Build history of the part. All positions in model axes, mm. A direction names the side the tool comes from. Round coordinates to 2 decimals unless told otherwise and drop trailing zeros. Order: outer loops, then holes, each group sorted by start corner. A loop starts at its lowest first (then second) coordinate and runs counter-clockwise, first axis right, second up. Notation, with made-up numbers: (28, 43.5) -> (41, 43.5) arc R31 ccw to (41, 72.5) -> close; hole circle Ø8 at (3, -35). An arc over 180 degrees is marked (long way). Use a Markdown table: item, result. Add a question column.
Item 1: Pin check, flat tip, straight feed: pin 1 (5 mm diameter, centred on x = 0, z = 0, fed in from -Y). Stop position of the tip, or through.
Item 2: 3-axis set-ups, long thin cutter, end or side, ignore diameter. For faces 4 (the face through (-16.9, -4.57, 0.18)), 5 (the face through (-1.86, -19.454, -7.746)): which of +Z, -Z, +X, -X, +Y, -Y reach the whole face in a straight line?
Item 3: Probe L1, parallel to Z at x = 0, y = -11; L2, parallel to X at y = -5, z = 5; L3, parallel to X at y = -6, z = -2.75. List the from-to ranges inside material, lowest first.
Item 4: Slice it at D-D, the plane x = -14. Give the cut face in (y, z), plus the area to 3 significant figures.
Item 5: Slice it at B-B, the plane y = -7. Give the cut face in (x, z), plus the area to 3 significant figures.
Item 6: Slice it at A-A, the plane z = 2.75. Give the cut face in (x, y).
Item 7: Slice it at C-C, the plane z = -10. Give the cut face in (x, y), plus the area to 3 significant figures.
Item 8: Two-plate mould, pull along X, no slides. Class faces 1 (the face through (0.61, -18.95, 8.21)), 2 (the face through (0, -10, -12.5)), 3 (the face through (-17.5, -8, 0)): released by +X, released by -X, zero draft, split by the parting line, or undercut.
from build123d import *

# Parameters (mm, degrees)
PAD_DEPTH         = 12.5
SKETCH001_R       = 4
POCKET_DEPTH      = 0.001
POCKET_DEPTH_BACK = -19.523712


with BuildPart() as part:
    # Sketch → Pad (new body, symmetric)
    with BuildSketch(Plane.XY):
        with BuildLine():
            ThreePointArc((-17.222222, -10.168336), (-11.903544, -16.07189), (-4.705882, -19.438484))
            ThreePointArc((-4.705882, -19.438484), (-4.355445, -19.50158), (-4, -19.522712))
            Line((-4, -19.522712), (-2.5, -19.522712))
            ThreePointArc((-2.5, -19.522712), (-1.850681, -19.4516), (-1.232145, -19.241635))
            Line((-1.232145, -19.241635), (0, -18.667076))
            Line((0, -18.667076), (1.232145, -19.241635))
            ThreePointArc((1.232145, -19.241635), (1.850681, -19.4516), (2.5, -19.522712))
            Line((2.5, -19.522712), (4, -19.522712))
            ThreePointArc((4, -19.522712), (4.355445, -19.50158), (4.705882, -19.438484))
            ThreePointArc((4.705882, -19.438484), (11.903544, -16.07189), (17.222222, -10.168336))
            ThreePointArc((17.222222, -10.168336), (17.429306, -9.678549), (17.5, -9.151503))
            Line((17.5, -9.151503), (17.5, -6))
            ThreePointArc((17.5, -6), (16.914214, -4.585786), (15.5, -4))
            Line((-15.5, -4), (15.5, -4))
            ThreePointArc((-15.5, -4), (-16.914214, -4.585786), (-17.5, -6))
            Line((-17.5, -9.151503), (-17.5, -6))
            ThreePointArc((-17.5, -9.151503), (-17.429306, -9.678549), (-17.222222, -10.168336))
        make_face()
    extrude(amount=PAD_DEPTH, both=True)

    # Sketch001 → Pocket (cut, two sides)
    with BuildSketch(Plane.XZ) as pocket_sk:
        Circle(SKETCH001_R)
    extrude(amount=-POCKET_DEPTH, mode=Mode.SUBTRACT)
    extrude(pocket_sk.sketch, amount=-POCKET_DEPTH_BACK, mode=Mode.SUBTRACT)


solid = part.part
Check sheet entries:
| question | item | result |
|---|---|---|
| 1 | pin 1 | through |
| 2 | face 4 | +Z, -Z, -X, +Y |
| 2 | face 5 | +Z, -Z, -Y |
| 3 | L1 | -12.5 to -4, 4 to 12.5 |
| 3 | L2 | -17.23 to 17.23 |
| 3 | L3 | -17.5 to -2.9, 2.9 to 17.5 |
| 4 | outline | (-14.28, -12.5) -> (-4, -12.5) -> (-4, 12.5) -> (-14.28, 12.5) -> close |
| 4 | area | 257 mm2 |
| 5 | outline | (-17.5, -12.5) -> (17.5, -12.5) -> (17.5, 12.5) -> (-17.5, 12.5) -> close; hole circle Ø8 at (0, 0) |
| 5 | area | 825 mm2 |
| 6 | outline | (-17.5, -9.15) arc R2 ccw to (-17.22, -10.17) arc R20 ccw to (-4.71, -19.44) arc R3 ccw to (-4, -19.52) -> (-2.9, -19.52) -> (-2.9, -4) -> (-15.5, -4) arc R2 ccw to (-17.5, -6) -> close; (2.9, -19.52) -> (4, -19.52) arc R3 ccw to (4.71, -19.44) arc R20 ccw to (17.22, -10.17) arc R2 ccw to (17.5, -9.15) -> (17.5, -6) arc R2 ccw to (15.5, -4) -> (2.9, -4) -> close |
| 7 | outline | (-17.5, -9.15) arc R2 ccw to (-17.22, -10.17) arc R20 ccw to (-4.71, -19.44) arc R3 ccw to (-4, -19.52) -> (-2.5, -19.52) arc R3 ccw to (-1.23, -19.24) -> (0, -18.67) -> (1.23, -19.24) arc R3 ccw to (2.5, -19.52) -> (4, -19.52) arc R3 ccw to (4.71, -19.44) arc R20 ccw to (17.22, -10.17) arc R2 ccw to (17.5, -9.15) -> (17.5, -6) arc R2 ccw to (15.5, -4) -> (-15.5, -4) arc R2 ccw to (-17.5, -6) -> close |
| 7 | area | 449 mm2 |
| 8 | face 1 | undercut |
| 8 | face 2 | zero draft |
| 8 | face 3 | released by -X |
